Check sheet for the drawn part. Datum: minimum x, y, z corner. Units: mm. Give positions to 0.01 mm unless a question says otherwise; leave off trailing zeros. Order: outer loops, then holes, each group sorted by start corner. A loop starts at its lowest first (then second) coordinate and runs counter-clockwise, first axis right, second up. Notation, with made-up numbers: M 27,48.25 L 82,48.25 A25 cw 82,74.25 Z; hole C 29.25,0 d6. An arc over 180 degrees is marked long. Put each result on its own line as item: value. Start each with the question number.
Q1. Go/stop test with flat-tipped pins: pin 1 (15 mm diameter, centred on x = 988, z = 176.5, fed in from +Y); pin 2 (6 mm diameter, centred on x = 442, y = 106.5, fed in from -Z); pin 3 (15 mm diameter, centred on x = 13.5, z = 212.5, fed in from -Y). Record where each tip stops, or that it passes through.
Q2. Section check B-B on y = 496.5. Record the cut outline in (x, z), then the cut area to 3 significant figures.
Q3. Material ranges on L1, parallel to Z at x = 801.5, y = 350; L2, parallel to Y at x = 519.5, z = 230; L3, parallel to Y at x = 973.5, z = 268.5, recorded low to high.
Q4. Section check A-A on z = 234. Record the cut outline in (x, y), then the cut area to 3 significant figures.
Q5. Section check D-D on x = 657.5. Record the cut outline in (y, z), then the cut area to 3 significant figures.
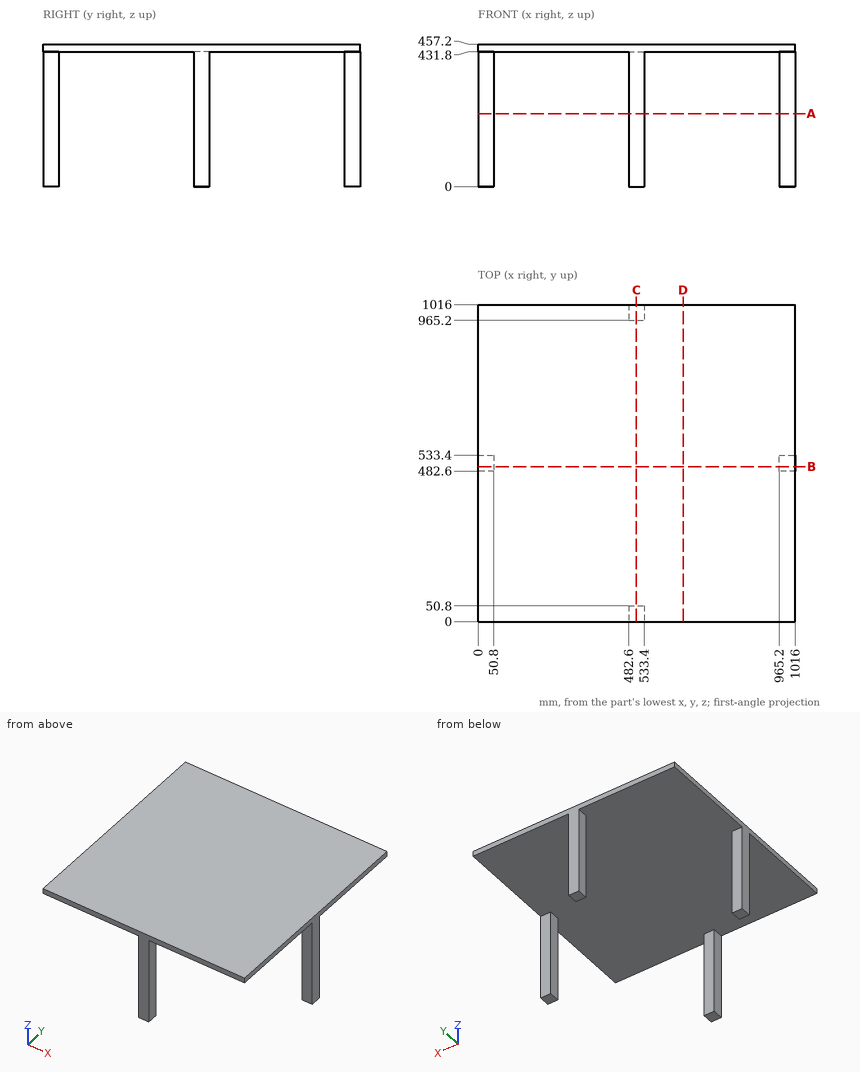
Results found:
1. pin 1: stops at y = 533.4
1. pin 2: stops at z = 431.8
1. pin 3: stops at y = 482.6
2. outline: M 0,0 L 50.8,0 L 50.8,431.8 L 965.2,431.8 L 965.2,0 L 1016,0 L 1016,457.2 L 0,457.2 Z
2. area: 69,700 mm^2
3. L1: z = 431.8 to 457.2
3. L2: y = 0 to 50.8, 965.2 to 1016
3. L3: y = 482.6 to 533.4
4. outline: M 0,482.6 L 50.8,482.6 L 50.8,533.4 L 0,533.4 Z; M 482.6,0 L 533.4,0 L 533.4,50.8 L 482.6,50.8 Z; M 482.6,965.2 L 533.4,965.2 L 533.4,1016 L 482.6,1016 Z; M 965.2,482.6 L 1016,482.6 L 1016,533.4 L 965.2,533.4 Z
4. area: 10,300 mm^2
5. outline: M 0,431.8 L 1016,431.8 L 1016,457.2 L 0,457.2 Z
5. area: 25,800 mm^2
